from build123d import *

# Parameters (mm, degrees)
CUT_EXTRUDE1_DEPTH = 2


with BuildPart() as part:
    # Sketch1 → Revolve1 (revolve)
    with BuildSketch(Plane.XY):
        Polygon((5, 0), (5, -1.75), (4.25, -2.5), (0.283190307, -2.5), (0, -2.0095), (0, -1.443375673), (0.833333333, 0), align=None)
    revolve(axis=Axis((0.833333333, 0, 0), (1, 0, 0)))

    # Sketch2 → Cut-Extrude1 (cut)
    with BuildSketch(Plane(origin=(0, 0, 0), x_dir=(0, 0, -1), z_dir=(1, 0, 0))):
        Polygon((-1.443375673, 0), (-0.721687836, -1.25), (0.721687836, -1.25), (1.443375673, 0), (0.721687836, 1.25), (-0.721687836, 1.25), align=None)
    extrude(amount=CUT_EXTRUDE1_DEPTH, mode=Mode.SUBTRACT)


solid = part.part
Design review of the part built by this model. Coordinates are the model's own, in mm. A direction names the side the tool comes from. Round coordinates to 2 decimals unless told otherwise and drop trailing zeros. Order: outer loops, then holes, each group sorted by start corner. A loop starts at its lowest first (then second) coordinate and runs counter-clockwise, first axis right, second up. Notation, with made-up numbers: M 50.5,70 L 91.5,70 A16 cw 91.5,93 Z; hole C -39,-7 d6. An arc over 180 degrees is marked long. Answer as CSV lines item,"result". Start each with the question number.
1) Wall thickness on line 1 along X through (y, z) = (0.7, 0.75); line 2 along Y through (x, z) = (0.7, 0.35); line 3 along Y through (x, z) = (1.4, 1): over which ranges is each line inside the solid? List them lowest first. Write a range as [from, to].
2) Add section C-C (x = 3). Give the boundary of the cut face in (y, z).
3) Tool access review of faces 4 (the face through (1, -1.25, 0)), 5 (the face through (0, 0.92, 1.31)): name each direction out of +Z, -Z, +X, -X, +Y, -Y from which nothing blocks a thin tool from reaching the whole face with its end or side.
4) For pin 1 Ø1 at (y, z) = (2, 1.5) entering from +X; pin 2 Ø1.5 at (x, y) = (2, 1.5) entering from -Z; pin 3 Ø0.8 at (y, z) = (0.5, -0.5) entering from -X, all flat-tipped, find the tip position at first contact; note any pin that passes through.
5) Add section A-A (x = 0.4). Give the boundary of the cut face in (y, z), then the cut area to 3 significant figures.
6) The part is to be moulded in two halves that separate along Y. For faces 1 (the face through (5, 0, 0)), 2 (the face through (2.24, 0.54, 2.44)), 3 (the face through (2, 0, 0)), say which applies: +Y half, -Y half, draft (parallel to the pull), parting line (faces both ways), or undercut.
7) Add section B-B (z = 0). Give the boundary of the cut face in (x, y), then the cut area to 3 significant figures.
Resolved:
1,line 1,"[2, 5]"
1,line 2,"[-2.48, -1.25], [1.25, 2.48]"
1,line 3,"[-2.29, -0.77], [0.77, 2.29]"
2,outline,"C 0,0 d5"
3,face 4,"-X"
3,face 5,"+Z, -Z, -X, +Y, -Y"
4,pin 1,"x = 4.75"
4,pin 2,"z = -2.38"
4,pin 3,"x = 2"
5,outline,"C 0,0 d5; hole M -1.25,-0.72 L 0,-1.44 L 1.25,-0.72 L 1.25,0.72 L 0,1.44 L -1.25,0.72 Z"
5,area,"14.2 mm^2"
6,face 1,"draft"
6,face 2,"parting line"
6,face 3,"undercut"
7,outline,"M 0,-2.01 L 0.28,-2.5 L 4.25,-2.5 L 5,-1.75 L 5,1.75 L 4.25,2.5 L 0.28,2.5 L 0,2.01 L 0,1.44 L 0.11,1.25 L 2,1.25 L 2,-1.25 L 0.11,-1.25 L 0,-1.44 Z"
7,area,"19.3 mm^2"
